Source: CAD feature listing. Evaluate the final solid. Frame: model axes, mm. Face numbers are marked on the shaded views. A direction names the side the tool comes from. Round coordinates to 2 decimals unless told otherwise and drop trailing zeros. Loops run counter-clockwise (first coordinate to the right, second up) from the corner with the lowest first, then second, coordinate; pieces in that order, holes last. Notation, with made-up numbers: M 5,18.25 L 10,18.25 A5 cw 10,23.25 Z; hole C 5.25,35 d10. An arc over 180 degrees is marked long. Answer as a JSON object with one key per item and string values.
Autodesk Inventor part; units mm, degrees
ref_plane "Work Plane1" through (75, 5.75, 0) normal (0, 1, 0) x (1, 0, 0)
ref_plane "YZ Plane" through (0, 0, 0) normal (1, 0, 0) x (0, 1, 0)
ref_plane "XZ Plane" through (0, 0, 0) normal (0, 1, 0) x (-1, 0, 0)
sketch "Sketch1" plane through (0, 0, 0) normal (0, 0, 1) x (1, 0, 0)
  line L0 (-75, -10) -> (-95, -10)
  line L1 (-95, -10) -> (-95, 10)
  line L2 (-95, 10) -> (-75, 10)
  line L3 (-75, 10) -> (-75, -10)
  line L4 (-75, -10) -> (-95, 10) construction
  line L5 (-95, -10) -> (-75, 10) construction
  line L6 (95, -10) -> (75, -10)
  line L7 (75, -10) -> (75, 10)
  line L8 (75, 10) -> (95, 10)
  line L9 (95, 10) -> (95, -10)
  line L10 (95, -10) -> (75, 10) construction
  line L11 (75, -10) -> (95, 10) construction
  line L12 (-85, 0) -> (85, 0) construction
  point P0 (0, 0)
  point P1 (0, 0)
  dimension "d0" = 20
  dimension "d1" = 20
  dimension "d2" = 20
  dimension "d3" = 20
  dimension "d4" = 170
extrude "Extrusion1" add sketch "Sketch1" along normal blind 5
sketch "Sketch2" plane through (0, 0, 5) normal (0, 0, 1) x (1, 0, 0)
  line L0 (-75, 10) -> (-95, 10)
  line L1 (-95, 10) -> (-95, -10)
  line L2 (-95, -10) -> (-75, -10)
  line L3 (-75, -10) -> (-75, 10)
  line L4 (95, 10) -> (75, 10)
  line L5 (75, 10) -> (75, -10)
  line L6 (75, -10) -> (95, -10)
  line L7 (95, -10) -> (95, 10)
  line L8 (-95, 10) -> (95, 10)
  line L9 (95, 10) -> (95, -10)
  line L10 (95, -10) -> (-95, -10)
  line L11 (-95, -10) -> (-95, 10)
  point P0 (0, 0)
extrude "Extrusion2" add sketch "Sketch2" along normal blind 5
ref_plane "Work Plane1" through (75, 5.75, 0) normal (0, 1, 0) x (1, 0, 0)
sketch "Sketch4" plane through (95, -10, 0) normal (1, 0, 0) x (0, 0, -1)
  line L0 (0, 0) -> (0, 20)
  line L1 (0, 20) -> (-10, 20)
  line L2 (-10, 0) -> (-10, 20)
  line L3 (0, 0) -> (-10, 0)
  line L4 (-10, 20) -> (-20, 20)
  line L5 (-20, 20) -> (-40.8378, -98.1769)
  line L6 (-40.8378, -98.1769) -> (-10, -109.401)
  line L7 (0, 0) -> (0, 20)
  line L8 (-10, -109.401) -> (-10, 0)
  line L9 (-10, 0) -> (-10, 20)
  point P0 (0, 10)
  dimension "d14" = 100
  dimension "d15" = 100
  dimension "d16" = 120
  dimension "d17" = 20
extrude "Extrusion4" add sketch "Sketch4" against normal up to surface (190 mm away) contours L8 L6 L5 L4 L2
fillet "Fillet1" radius 2 2 edges at (-75, 0, 5) (75, 0, 5)
fillet "Fillet2" radius 1 9 edges at (-75, 10, 1.5) (75, 10, 1.5) (-75, -10, 1.5) (75, -10, 1.5) (95, -10, 5) (95, 10, 10) (-95, 10, 10) (-95, -10, 5) (95, -113.7889, 25.4189)
equation "\"d15\" = d14"
properties part number "Display Case" material "ABS Plastic"
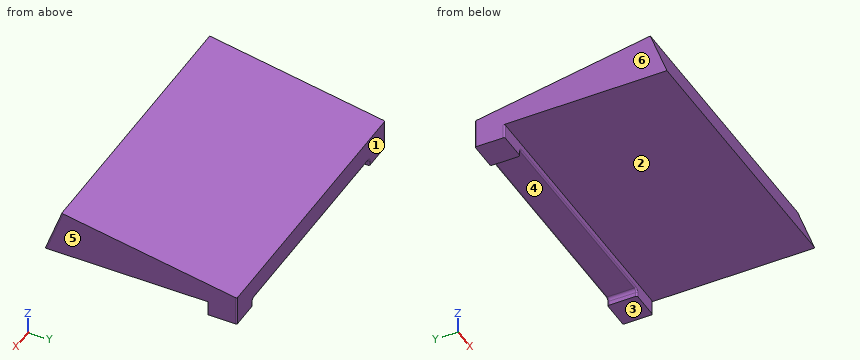
Item 1: Line query: probe 1 along Y at (x, z) = (11, 6); probe 2 along Z at (x, y) = (-33.5, -5); probe 3 along Z at (x, y) = (22, -65). Output: solid intervals per line, ascending. Write a range as from..to.
Answer sheet:
{"probe 1": "y = -10..10", "probe 2": "z = 5..22.64", "probe 3": "z = 10..33.22"}
Item 2: Pull-direction query (X, two-part tool) for the marked faces 3, 4, 5 and 6; classes: pulls with the +X half, pulls with the -X half, needs draft (parallel to the pull), parting line crosses it, or undercut.
Answer sheet:
{"face 3": "needs draft", "face 4": "undercut", "face 5": "pulls with the +X half", "face 6": "pulls with the -X half"}
Item 3: Access query for the marked faces 1 and 2. Directions: +Z, -Z, +X, -X, +Y, -Y. A direction counts if a zero-diameter tool reaches every point of the face in a straight line with its end or side. Return the directions, or none.
Answer sheet:
{"face 1": "+Z, -Z, +X, -X, +Y", "face 2": "-Z, +X, -X, -Y"}
Item 4: Section B-B on y = -43.5. Return the cut outline in (x, z), then the cut area to 3 significant figures.
Answer sheet:
{"outline": "M -95,10 L 95,10 L 95,29.43 L -95,29.43 Z", "area": "3,690 mm²"}
Item 5: Contact query for flat-ended pins moving along their axis: pin 1 Ø12 at (x, y) = (-25.5, -44.5) entering from +Z; pin 2 Ø6 at (x, y) = (45.5, -99.5) entering from -Z; pin 3 Ø12 at (x, z) = (12, 36) entering from -Y. Output: stop coordinate, or through.
Answer sheet:
{"pin 1": "stops at z = 30.67", "pin 2": "stops at z = 10", "pin 3": "stops at y = -112.12"}
Item 6: Section C-C on y = -103. Return the cut outline in (x, z).
Answer sheet:
{"outline": "M -95,10 L 95,10 L 95,39.92 L -95,39.92 Z"}
Item 7: Section A-A on x = 62.5. Return the cut outline in (y, z).
Answer sheet:
{"outline": "M -119.4,10 L -10,10 L -10,6 A1 ccw -9,5 L 9,5 A1 ccw 10,6 L 10,20 L -108.18,40.84 Z"}
